Build history of the part. All positions in model axes, mm. A direction names the side the tool comes from. Round coordinates to 2 decimals unless told otherwise and drop trailing zeros. Loops run counter-clockwise (first coordinate to the right, second up) from the corner with the lowest first, then second, coordinate; pieces in that order, holes last.
Autodesk Inventor part; units mm, degrees
ref_plane "YZ Plane" through (0, 0, 0) normal (1, 0, 0) x (0, 1, 0)
ref_plane "XZ Plane" through (0, 0, 0) normal (0, 1, 0) x (-1, 0, 0)
ref_plane "XY Plane" through (0, 0, 0) normal (0, 0, 1) x (1, 0, 0)
sketch "Sketch1" plane through (0, 0, 0) normal (0, 1, 0) x (-1, 0, 0)
  line L0 (-40, 27.5) -> (40, 27.5)
  line L1 (40, 27.5) -> (40, -27.5)
  line L2 (40, -27.5) -> (-40, -27.5)
  line L3 (-40, -27.5) -> (-40, 27.5)
  line L4 (-40, 27.5) -> (40, -27.5) construction
  line L5 (40, 27.5) -> (-40, -27.5) construction
  line L6 (40, 27.5) -> (43, 27.5)
  line L7 (43, 27.5) -> (43, -27.5)
  line L8 (43, -27.5) -> (40, -27.5)
  line L9 (40, -27.5) -> (40, 27.5)
  line L10 (-40, 27.5) -> (-43, 27.5)
  line L11 (-43, 27.5) -> (-43, -27.5)
  line L12 (-43, -27.5) -> (-40, -27.5)
  line L13 (-40, -27.5) -> (-40, 27.5)
  point P0 (0, 0)
  point P1 (-40, -27.5)
  dimension "d0" = 80
  dimension "d1" = 55
  dimension "d2" = 3
  dimension "d3" = 3
extrude "Extrusion1" add sketch "Sketch1" along normal blind 3 contours L0 L1 L2 L3
extrude "Extrusion2" add sketch "Sketch1" along normal blind 63 contours L3 L12 L11 L10 | L6 L7 L8 L1
sketch "Sketch2" plane through (0, 3, 0) normal (0, 1, 0) x (1, 0, 0)
  line L0 (12.875, -7.5) -> (-12.875, -7.5)
  line L1 (-12.875, -7.5) -> (-12.875, 7.5)
  line L2 (-12.875, 7.5) -> (12.875, 7.5)
  line L3 (12.875, 7.5) -> (12.875, -7.5)
  line L4 (12.875, -7.5) -> (-12.875, 7.5) construction
  line L5 (-12.875, -7.5) -> (12.875, 7.5) construction
  line L6 (12.875, 7.5) -> (17.125, 7.5)
  circle A0 centre (15, 7.5) radius 2.125
  circle A1 centre (15, -7.5) radius 2.125
  line L7 (-12.875, -7.5) -> (-17.125, -7.5)
  circle A2 centre (-15, -7.5) radius 2.125
  circle A3 centre (-15, 7.5) radius 2.125
  point P0 (0, 0)
  dimension "d8" = 25.75
  dimension "d9" = 15
  dimension "d10" = 4.25
  dimension "d11" = 4.25
extrude "Extrusion3" cut sketch "Sketch2" against normal through all contours A2 L7 | L7 A2 | A3 | A0 L6 | L6 A0 | A1
sketch "Sketch3" plane through (-43, 0, -27.5) normal (-1, 0, 0) x (0, 0, 1)
  circle A0 centre (27.5, 34) radius 4.5
  line L0 (0, 0) -> (55, 0)
  circle A1 centre (27.5, 34) radius 29
  line L1 (0, 3) -> (0, 63)
  line L2 (0, 43.206) -> (0, 63)
  line L3 (0, 63) -> (27.5, 63)
  line L4 (55, 63) -> (0, 63)
  line L5 (27.5, 63) -> (55, 63)
  line L6 (55, 63) -> (55, 43.206)
  line L7 (55, 3) -> (55, 63)
  point P0 (27.5, 0)
  dimension "d14" = 9
  dimension "d15" = 34
extrude "Extrusion4" cut sketch "Sketch3" against normal through all contours A0
extrude "Extrusion5" cut sketch "Sketch3" against normal through all contours A1 L4 L6 | A1 L1 L3
properties part number "baseatas2" material "Aluminum 6061"
(1) Pin check, flat tips, straight feed: P1, Ø3.5, axis at x = 15, z = -7.5, coming from the -Y side; P2, Ø5, axis at x = -15, z = -7.5, coming from the +Y side. Stop position of each tip, or through.
Responses:
P1: passes through
P2: stops at y = 3
(2) Slice it at B-B on x = 15. List the corners of the cut face in (y, z) (3 decimals), plus the area to 4 significant figures.
Responses:
outline: (0, -27.5) - (3, -27.5) - (3, -9.625) - (0, -9.625) - close; (0, -5.375) - (3, -5.375) - (3, 5.375) - (0, 5.375) - close; (0, 9.625) - (3, 9.625) - (3, 27.5) - (0, 27.5) - close
area: 139.5 mm2
(3) Pull direction X, two halves, no side cores. Call faces 3 (the face through (41.48, 29.61, -0.98)), 4 (the face through (43, 24, 0)), 5 (the face through (1, 3, 0)): +X half, -X half, draft (parallel to the pull), parting line (faces both ways), or undercut.
Responses:
face 3: draft
face 4: +X half
face 5: undercut
(4) Slice it at C-C on z = -7.5. List the corners of the cut face in (x, y) (3 decimals).
Responses:
outline: (-43, 0) - (-17.125, 0) - (-17.125, 3) - (-40, 3) - (-40, 62.013) - (-43, 62.013) - close; (-12.875, 0) - (12.875, 0) - (12.875, 3) - (-12.875, 3) - close; (17.125, 0) - (43, 0) - (43, 62.013) - (40, 62.013) - (40, 3) - (17.125, 3) - close
(5) Probe line 1 (Z direction, x = 15, y = 1.9) (3 decimals); line 2 (X direction, y = 1.4, z = -7.5) (3 decimals); line 3 (X direction, y = 57, z = 12.5). List the from-to ranges inside material, lowest first.
Responses:
line 1: z = -27.5 to -9.625, -5.375 to 5.375, 9.625 to 27.5
line 2: x = -43 to -17.125, -12.875 to 12.875, 17.125 to 43
line 3: x = -43 to -40, 40 to 43
(6) Slice it at A-A on y = 24. List the corners of the cut face in (x, z).
Responses:
outline: (-43, -27.5) - (-40, -27.5) - (-40, 27.5) - (-43, 27.5) - close; (40, -27.5) - (43, -27.5) - (43, 27.5) - (40, 27.5) - close
(7) Which spindle directions (+Z, -Z, +X, -X, +Y, -Y) get a long thin tool onto all of the face, cutting with end or side? Do faces 1 (the face through (-40, 26, 0)), 2 (the face through (-43, 24, 0)). Say none if no direction does.
Responses:
face 1: +Z, -Z, +Y
face 2: +Z, -Z, -X, +Y, -Y
(8) Slice it at D-D on y = 53.5. List the corners of the cut face in (x, z), plus the area to 3 significant figures.
Responses:
outline: (-43, -21.47) - (-40, -21.47) - (-40, 21.47) - (-43, 21.47) - close; (40, -21.47) - (43, -21.47) - (43, 21.47) - (40, 21.47) - close
area: 258 mm2
